Verification items for the finished model (mm, model axes). Give positions to 0.01 mm unless a question says otherwise; leave off trailing zeros. Order: outer loops, then holes, each group sorted by start corner. A loop starts at its lowest first (then second) coordinate and runs counter-clockwise, first axis right, second up. Notation, with made-up numbers: M 21.25,81 L 67.25,81 A37 cw 67.25,117 Z; hole C -23,16 d8. An arc over 180 degrees is marked long. Answer as a JSON object with one key per item and string values.
```python
from build123d import *

# Parameters (mm, degrees)
F0_W        = 177.8
F0_H        = 12.7
F1_DEPTH    = 12.7
F2_T1_DEPTH = 76.2


# Not quite as in the source:
# - a fillet or chamfer that OpenCascade refuses, or shapes differently, is made with other operations: its cross-section is extruded or revolved along the edge and cut away or added


with BuildPart() as f1:
    # F0 (on Front) → F1 (new body)
    with BuildSketch(Plane.XZ):
        with Locations((21.4704718173, 53.7259025425)):
            Rectangle(F0_W, F0_H)
    extrude(amount=F1_DEPTH)

    # F2: fillet of radius 12.7 on 4 edges, made by hand

    # F2_s2 → F2_t1 (cut)
    with BuildSketch(Plane.XZ.offset(-31.75)):
        with BuildLine():
            ThreePointArc((-67.4295281827, 47.3759025425), (-63.7097843038, 56.3561586636), (-54.7295281827, 60.0759025425))
            Line((-54.7295281827, 60.0759025425), (-67.4295281827, 60.0759025425))
            Line((-67.4295281827, 60.0759025425), (-67.4295281827, 47.3759025425))
        make_face()
        with BuildLine():
            ThreePointArc((110.3704718173, 47.3759025425), (106.6507279383, 56.3561586636), (97.6704718173, 60.0759025425))
            Line((97.6704718173, 60.0759025425), (110.3704718173, 60.0759025425))
            Line((110.3704718173, 60.0759025425), (110.3704718173, 47.3759025425))
        make_face()
        with BuildLine():
            ThreePointArc((97.6704718173, 47.3759025425), (106.6507279383, 51.0956464214), (110.3704718173, 60.0759025425))
            Line((110.3704718173, 60.0759025425), (110.3704718173, 47.3759025425))
            Line((110.3704718173, 47.3759025425), (97.6704718173, 47.3759025425))
        make_face()
        with BuildLine():
            ThreePointArc((-67.4295281827, 60.0759025425), (-63.7097843038, 51.0956464214), (-54.7295281827, 47.3759025425))
            Line((-54.7295281827, 47.3759025425), (-67.4295281827, 47.3759025425))
            Line((-67.4295281827, 47.3759025425), (-67.4295281827, 60.0759025425))
        make_face()
    extrude(amount=F2_T1_DEPTH, mode=Mode.SUBTRACT)


solid = f1.part
```
Q1. Section check B-B on z = 50.5. Record the cut outline in (x, y), then the cut area to 3 significant figures.
Resolved:
{"outline": "M -63.07,-12.7 L 106.01,-12.7 L 106.01,0 L -63.07,0 Z", "area": "2,150 mm²"}
Q2. Section check C-C on z = 57.75. Record the cut outline in (x, y), then the cut area to 3 significant figures.
Resolved:
{"outline": "M -62.06,-12.7 L 105,-12.7 L 105,0 L -62.06,0 Z", "area": "2,120 mm²"}
Q3. Material ranges on L1, parallel to X at y = -2.25, z = 53.75; L2, parallel to X at y = -9, z = 52.25, recorded low to high.
Resolved:
{"L1": "x = -65.71 to 108.66", "L2": "x = -64.73 to 107.67"}
Q4. Gauge pin test, flat ends, axial feed: pin 1 Ø1.5 at (y, z) = (-1.5, 51) entering from -X; pin 2 Ø2 at (y, z) = (-10, 57) entering from -X; pin 3 Ø5 at (y, z) = (-9.5, 50) entering from +X. Record the tip position at first contact, or that the pin passes through.
Resolved:
{"pin 1": "stops at x = -64.32", "pin 2": "stops at x = -64.05", "pin 3": "stops at x = 107.86"}
Q5. Section check A-A on y = -2.25. Record the cut outline in (x, z), then the cut area to 3 significant figures.
Resolved:
{"outline": "M -65.73,53.73 A12.7 ccw -54.73,47.38 L 97.67,47.38 A12.7 ccw 108.67,53.73 A12.7 ccw 97.67,60.08 L -54.73,60.08 A12.7 ccw Z", "area": "2,130 mm²"}
